The model under review builds one solid part; all positions refer to its coordinate system, in mm. A direction names the side the tool comes from. Round coordinates to 2 decimals unless told otherwise and drop trailing zeros. Write each loop counter-clockwise with the first axis right and the second up, starting at its lowest first coordinate (ties: lowest second). Pieces come first, ordered by that corner, then holes.
Item 1: Add section B-B (x = 62). Give the boundary of the cut face in (y, z), plus the area to 3 significant figures.
Item 2: Add section D-D (z = -19). Give the boundary of the cut face in (x, y), plus the area to 3 significant figures.
Item 3: Clearance check with flat-ended pins moving along their axes: pin 1 Ø4 at (x, y) = (82, 1) entering from +Z; pin 2 Ø5 at (x, y) = (81.5, 4.5) entering from +Z; pin 3 Ø3 at (y, z) = (5.5, -30.5) entering from +X. State where each tip first meets the part, or that it passes through.
Item 4: Add section A-A (z = -28). Give the boundary of the cut face in (x, y).
Item 5: Machinability: for faces 1 (the face through (64, 5, -24)), 2 (the face through (79.83, 4.93, -34.88)), which of the approach directions +Z, -Z, +X, -X, +Y, -Y give a long, thin tool a straight path to every point of the face, cutting with its end or side? Answer none if there is none.
Item 6: To check wall thickness, follow L1, parallel to Z at x = 60.5, y = 3.25; L2, parallel to X at y = 2, z = -28; L3, parallel to X at y = 2.5, z = -10.5. State the ranges of each line that lie inside material, in increasing order.
Item 7: Add section C-C (y = 6). Give the boundary of the cut face in (x, z), plus the area to 3 significant figures.
```python
from build123d import *

# Parameters (mm, degrees)
BOSS_EXTRUDE1_DEPTH = 10


with BuildPart() as part:
    # Sketch1 → Boss-Extrude1 (new body)
    with BuildSketch(Plane(origin=(0, 0, 0), x_dir=(1, 0, 0), z_dir=(0, 1, 0))):
        with BuildLine():
            Line((50, 0), (50, 40))
            Line((50, 40), (70, 40))
            ThreePointArc((70, 40), (79.926416645, 34.742866793), (81.155417528, 23.577708764))
            ThreePointArc((81.155417528, 23.577708764), (89.893958659, 10.408225074), (78, 0))
            Line((78, 0), (50, 0))
        make_face()
        with BuildLine():
            Line((58, 32), (58, 24))
            Line((58, 24), (70, 24))
            ThreePointArc((70, 24), (74, 28), (70, 32))
            Line((70, 32), (58, 32))
        make_face(mode=Mode.SUBTRACT)
        with BuildLine():
            Line((58, 8), (78, 8))
            ThreePointArc((78, 8), (82, 12), (78, 16))
            Line((78, 16), (58, 16))
            Line((58, 16), (58, 8))
        make_face(mode=Mode.SUBTRACT)
    extrude(amount=BOSS_EXTRUDE1_DEPTH)


solid = part.part
```
Numbers:
1. outline: (0, -40) - (10, -40) - (10, -32) - (0, -32) - close; (0, -24) - (10, -24) - (10, -16) - (0, -16) - close; (0, -8) - (10, -8) - (10, 0) - (0, 0) - close
1. area: 240 mm2
2. outline: (50, 0) - (87.75, 0) - (87.75, 10) - (50, 10) - close
2. area: 377 mm2
3. pin 1: stops at z = -0.17
3. pin 2: stops at z = -0.04
3. pin 3: stops at x = 81.96
4. outline: (50, 0) - (58, 0) - (58, 10) - (50, 10) - close; (74, 0) - (82, 0) - (82, 10) - (74, 10) - close
5. face 1: +Y, -Y
5. face 2: +X, +Y, -Y
6. L1: z = -40 to -32, -24 to -16, -8 to 0
6. L2: x = 50 to 58, 74 to 82
6. L3: x = 50 to 58, 81.71 to 89.91
7. outline: (50, -40) - (70, -40) arc R12 ccw to (81.16, -23.58) arc R12 ccw to (78, 0) - (50, 0) - close; hole (58, -32) - (70, -32) arc R4 ccw to (70, -24) - (58, -24) - close; hole (58, -16) - (78, -16) arc R4 ccw to (78, -8) - (58, -8) - close
7. area: 1,070 mm2
